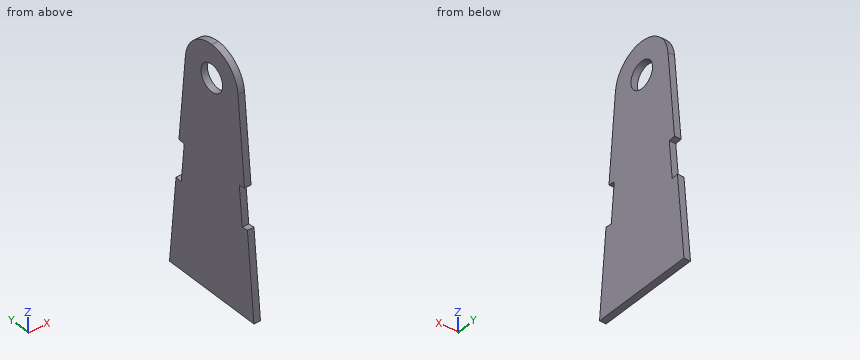
```python
from build123d import *

# Parameters (mm, degrees)
BOSS_EXTRUDE1_DEPTH     = 1.5875
F_1_4_CLEARANCE_HOLE1_D = 6.5278


with BuildPart() as part:
    # Sketch1 → Boss-Extrude1 (new body)
    with BuildSketch(Plane(origin=(0, 0, 0), x_dir=(0, 0, -1), z_dir=(1, 0, 0))):
        with BuildLine():
            ThreePointArc((-0.735600854, 7.903340916), (-5.86697273, 5.346263858), (-7.9375, 0))
            Line((-7.9375, 0), (50.8, 0))
            Line((50.8, 0), (50.8, 12.7))
            Line((50.8, 12.7), (29.774204123, 10.74303097))
            Line((29.774204123, 10.74303097), (29.921324293, 9.162362787))
            Line((29.921324293, 9.162362787), (20.437315194, 8.279641762))
            Line((20.437315194, 8.279641762), (20.290195023, 9.860309946))
            Line((20.290195023, 9.860309946), (-0.735600854, 7.903340916))
        make_face()
        with BuildLine():
            ThreePointArc((-7.9375, 0), (-5.86697273, -5.346263858), (-0.735600854, -7.903340916))
            Line((-0.735600854, -7.903340916), (20.290195023, -9.860309946))
            Line((20.290195023, -9.860309946), (20.437315194, -8.279641762))
            Line((20.437315194, -8.279641762), (29.921324293, -9.162362787))
            Line((29.921324293, -9.162362787), (29.774204123, -10.74303097))
            Line((29.774204123, -10.74303097), (50.8, -12.7))
            Line((50.8, -12.7), (50.8, 0))
            Line((50.8, 0), (-7.9375, 0))
        make_face()
    extrude(amount=BOSS_EXTRUDE1_DEPTH)

    # 1/4 Clearance Hole1 (through all)
    with Locations(Plane(origin=(1.5875, 0, 0), x_dir=(0, 0, -1), z_dir=(1, 0, 0))):
        with Locations((0, 0)):
            Hole(F_1_4_CLEARANCE_HOLE1_D / 2)


solid = part.part
```
Can you work these out from the model? Positions are in its coordinate system, mm. Round coordinates to 2 decimals unless told otherwise and drop trailing zeros. Loops run counter-clockwise (first coordinate to the right, second up) from the corner with the lowest first, then second, coordinate; pieces in that order, holes last. Notation, with made-up numbers: (-17.5, 30.5) -> (7.5, 30.5) arc R21 cw to (7.5, 51.5) -> close; hole circle Ø6 at (74.25, 0.25). An arc over 180 degrees is marked (long way). One line per item, written item: value. Start each with the question number.
1. If we section it at A-A, the plane x = 0.9: Write out the boundary of the cut face in (y, z) (1 decimal).
2. If I drill on probe 1 along Z at (x, y) = (0.2, 0.5); probe 2 along Y at (x, z) = (0.95, 2.5); probe 3 along Y at (x, z) = (1.35, 0), over which ranges is the centre line in solid material (lowest first)?
3. If we section it at D-D, the plane z = -41: Write out the boundary of the cut face in (x, y).
4. If we section it at C-C, the plane y = 5.25: Write out the boundary of the cut face in (x, z), then the cut area to 3 significant figures.
5. If we section it at B-B, the plane z = 0: Write out the boundary of the cut face in (x, y).
6. For pin 1 (5 mm diameter, centred on y = 0, z = 0, fed in from +X), with a flat end and sliding along its axis, tell me the tip position at first contact or that it passes through.
Calculated:
1. outline: (-12.7, -50.8) -> (12.7, -50.8) -> (10.7, -29.8) -> (9.2, -29.9) -> (8.3, -20.4) -> (9.9, -20.3) -> (7.9, 0.7) arc R7.9 ccw to (-7.9, 0.7) -> (-9.9, -20.3) -> (-8.3, -20.4) -> (-9.2, -29.9) -> (-10.7, -29.8) -> close; hole circle Ø6.5 at (0, 0)
2. probe 1: z = -50.8 to -3.23, 3.23 to 7.92
2. probe 2: y = -7.53 to -2.1, 2.1 to 7.53
2. probe 3: y = -7.97 to -3.26, 3.26 to 7.97
3. outline: (0, -11.79) -> (1.59, -11.79) -> (1.59, 11.79) -> (0, 11.79) -> close
4. outline: (0, -50.8) -> (1.59, -50.8) -> (1.59, 5.95) -> (0, 5.95) -> close
4. area: 90.1 mm²
5. outline: (0, -7.97) -> (1.59, -7.97) -> (1.59, -3.26) -> (0, -3.26) -> close; (0, 3.26) -> (1.59, 3.26) -> (1.59, 7.97) -> (0, 7.97) -> close
6. pin 1: passes through
